Can you work these out from the model? Positions are in its coordinate system, mm. A direction names the side the tool comes from. Give positions to 0.01 mm unless a question says otherwise; leave off trailing zeros. Write each loop counter-clockwise with the first axis right and the second up, starting at its lowest first coordinate (ties: lowest second). Pieces come first, ordered by that corner, then holes. Notation, with made-up numbers: (74, 36.5) -> (94, 36.5) arc R12 ccw to (94, 47.5) -> close; hole circle Ø8 at (10.25, -19.75). An arc over 180 degrees is marked (long way). Answer as CSV lines item,"result". Start each with the question number.
1. If we mould it in two halves opening along X, with no side actions, what happens to faces 1 (the face through (-79.15, 46.07, 0.74)), 2 (the face through (-1, 1, 1.5))? For each: pulls with the +X half, pulls with the -X half, needs draft (parallel to the pull), parting line crosses it, or undercut.
2. I'm going to push flat-ended pins straight in: P1, Ø2, axis at x = -77.45, y = 46, coming from the +Z side; P2, Ø0.8, axis at x = -30.5, z = -2, coming from the +Y side (3 decimals); P3, Ø10, axis at x = 29, y = 1.5, coming from the -Z side. Where does each tip first touch, or does it pass through?
3. If we section it at D-D on x = 59: Write out the boundary of the cut face in (y, z).
4. On a 3-axis mill with a long thin cutter (end or side, diameter ignored), from which of +Z, -Z, +X, -X, +Y, -Y can I reach the whole of each face in a straight line? I mean faces 3 (the face through (-1, 1, 0)), 4 (the face through (79.15, 45.93, 0.74)). Say none if no direction works.
5. If we section it at A-A on x = -77.45: Write out the boundary of the cut face in (y, z), plus the area to 3 significant figures.
6. If we section it at C-C on y = -19: Write out the boundary of the cut face in (x, z), plus the area to 3 significant figures.
7. I need wall thicknesses on line 1 (Y direction, x = -77.45, z = 0.6); line 2 (Y direction, x = -77.45, z = 0.45); line 3 (Y direction, x = -11.5, z = -1.75). Which ranges of each line are inside material? Lowest first, please. Write a range as [from, to].
8. If we section it at B-B on y = 46: Write out the boundary of the cut face in (x, z), plus the area to 3 significant figures.
```python
from build123d import *

# Parameters (mm, degrees)
SKETCH1_W           = 165
SKETCH1_H           = 102.1
SKETCH1_R           = 1.7
BOSS_EXTRUDE1_DEPTH = 1.5
SKETCH2_W           = 172
SKETCH2_H           = 109.1
SKETCH2_W_2         = 165
SKETCH2_H_2         = 102.1
BOSS_EXTRUDE2_DEPTH = 4
SKETCH3_W           = 165
SKETCH3_H           = 1
CUT_EXTRUDE1_DEPTH  = 2.5
FILLET1_R           = 1


with BuildPart() as part:
    # Sketch1 → Boss-Extrude1 (new body)
    with BuildSketch(Plane.XY):
        Rectangle(SKETCH1_W, SKETCH1_H)
        with Locations((-77.45, 46)):
            Circle(SKETCH1_R, mode=Mode.SUBTRACT)
        with Locations(Location((77.45, 46, 0), (0, 0, 180))):
            Circle(SKETCH1_R, mode=Mode.SUBTRACT)
        with Locations((77.45, -46)):
            Circle(SKETCH1_R, mode=Mode.SUBTRACT)
        with Locations(Location((-77.45, -46, 0), (0, 0, 180))):
            Circle(SKETCH1_R, mode=Mode.SUBTRACT)
    extrude(amount=BOSS_EXTRUDE1_DEPTH)

    # Sketch2 → Boss-Extrude2 (add)
    with BuildSketch(Plane.XY.offset(1.5)):
        Rectangle(SKETCH2_W, SKETCH2_H)
        Rectangle(SKETCH2_W_2, SKETCH2_H_2, mode=Mode.SUBTRACT)
    extrude(amount=-BOSS_EXTRUDE2_DEPTH)

    # Sketch3 → Cut-Extrude1 (cut)
    with BuildSketch(Plane(origin=(0, 0, -2.5), x_dir=(-1, 0, 0), z_dir=(0, 0, -1))):
        with Locations((0, 51.55)):
            Rectangle(SKETCH3_W, SKETCH3_H)
    extrude(amount=-CUT_EXTRUDE1_DEPTH, mode=Mode.SUBTRACT)

    # Fillet1
    fillet1_edges = [part.edges().sort_by_distance(p)[0] for p in [
        (-86, 0, -2.5),
        (-86, -54.55, -0.5),
        (0, 54.55, -2.5),
        (-86, 54.55, -0.5),
        (86, 0, -2.5),
        (86, 54.55, -0.5),
        (0, -54.55, -2.5),
        (86, -54.55, -0.5),
        (-86, 0, 1.5),
        (0, -54.55, 1.5),
        (86, 0, 1.5),
        (0, 54.55, 1.5),
    ]]
    fillet(fillet1_edges, radius=FILLET1_R)


solid = part.part
```
Computed values:
1,face 1,"undercut"
1,face 2,"needs draft"
2,P1,"passes through"
2,P2,"stops at y = 54.545"
2,P3,"stops at z = 0"
3,outline,"(-54.55, -1.5) arc R1 ccw to (-53.55, -2.5) -> (-51.05, -2.5) -> (-51.05, 0) -> (52.05, 0) -> (52.05, -2.5) -> (53.55, -2.5) arc R1 ccw to (54.55, -1.5) -> (54.55, 0.5) arc R1 ccw to (53.55, 1.5) -> (-53.55, 1.5) arc R1 ccw to (-54.55, 0.5) -> close"
4,face 3,"-Z"
4,face 4,"+Z, -Z"
5,outline,"(-54.55, -1.5) arc R1 ccw to (-53.55, -2.5) -> (-51.05, -2.5) -> (-51.05, 0) -> (-47.7, 0) -> (-47.7, 1.5) -> (-53.55, 1.5) arc R1 ccw to (-54.55, 0.5) -> close; (-44.3, 0) -> (44.3, 0) -> (44.3, 1.5) -> (-44.3, 1.5) -> close; (47.7, 0) -> (52.05, 0) -> (52.05, -2.5) -> (53.55, -2.5) arc R1 ccw to (54.55, -1.5) -> (54.55, 0.5) arc R1 ccw to (53.55, 1.5) -> (47.7, 1.5) -> close"
5,area,"168 mm2"
6,outline,"(-86, -1.5) arc R1 ccw to (-85, -2.5) -> (-82.5, -2.5) -> (-82.5, 0) -> (82.5, 0) -> (82.5, -2.5) -> (85, -2.5) arc R1 ccw to (86, -1.5) -> (86, 0.5) arc R1 ccw to (85, 1.5) -> (-85, 1.5) arc R1 ccw to (-86, 0.5) -> close"
6,area,"275 mm2"
7,line 1,"y = [-54.54, -47.7], [-44.3, 44.3], [47.7, 54.54]"
7,line 2,"y = [-54.55, -47.7], [-44.3, 44.3], [47.7, 54.55]"
7,line 3,"y = [-54.52, -51.05], [52.05, 54.52]"
8,outline,"(-86, -1.5) arc R1 ccw to (-85, -2.5) -> (-82.5, -2.5) -> (-82.5, 0) -> (-79.15, 0) -> (-79.15, 1.5) -> (-85, 1.5) arc R1 ccw to (-86, 0.5) -> close; (-75.75, 0) -> (75.75, 0) -> (75.75, 1.5) -> (-75.75, 1.5) -> close; (79.15, 0) -> (82.5, 0) -> (82.5, -2.5) -> (85, -2.5) arc R1 ccw to (86, -1.5) -> (86, 0.5) arc R1 ccw to (85, 1.5) -> (79.15, 1.5) -> close"
8,area,"264 mm2"
